```python
from build123d import *

# Parameters (mm, degrees)
SKETCH1_R               = 7.25
SKETCH1_R_2             = 4.25
SKETCH1_W               = 3
SKETCH1_H               = 32
SKETCH1_W_2             = 32
SKETCH1_H_2             = 3
BOSS_EXTRUDE1_DEPTH     = 2
SKETCH1_3_R             = 7.25
SKETCH1_3_R_2           = 4.25
BOSS_EXTRUDE2_DEPTH     = 12
SKETCH5_W               = 9.5
SKETCH5_H               = 6.5
SKETCH5_W_2             = 5.5
SKETCH5_H_2             = 2.5
BOSS_EXTRUDE3_DEPTH     = 10
CUT_EXTRUDE1_DEPTH      = 47.818799643
CUT_EXTRUDE1_DEPTH_BACK = 47.818799643
SKETCH2_R               = 1.5
CUT_EXTRUDE3_DEPTH      = 47.818799643
CUT_EXTRUDE3_DEPTH_BACK = 47.818799643
SKETCH3_R               = 4.25


with BuildPart() as part:
    # Sketch1 → Boss-Extrude1 (new body)
    # profile 1 of 17: a face of its own
    with BuildSketch(Plane(origin=(0, 0, 0), x_dir=(1, 0, 0), z_dir=(0, 1, 0))):
        Circle(SKETCH1_R)
        Circle(SKETCH1_R_2, mode=Mode.SUBTRACT)
    # profile 2 of 17: a face of its own
    with BuildSketch(Plane(origin=(0, 0, 0), x_dir=(1, 0, 0), z_dir=(0, 1, 0))):
        Polygon((-0.461939766, 0.191341716), (11.783930069, 29.755486757), (14.555568667, 28.607436459), (2.309698831, -0.956708581), align=None)
    # profile 3 of 17: a face of its own
    with BuildSketch(Plane(origin=(0, 0, 0), x_dir=(1, 0, 0), z_dir=(0, 1, 0))):
        with Locations((1, 16)):
            Rectangle(SKETCH1_W, SKETCH1_H)
    # profile 4 of 17: a face of its own
    with BuildSketch(Plane(origin=(0, 0, 0), x_dir=(1, 0, 0), z_dir=(0, 1, 0))):
        Polygon((-0.353553391, 0.353553391), (22.273863607, 22.980970389), (24.395183951, 20.859650045), (1.767766953, -1.767766953), align=None)
    # profile 5 of 17: a face of its own
    with BuildSketch(Plane(origin=(0, 0, 0), x_dir=(1, 0, 0), z_dir=(0, 1, 0))):
        Polygon((-0.191341716, 0.461939766), (29.372803324, 12.707809602), (30.520853621, 9.936171004), (0.956708581, -2.309698831), align=None)
    # profile 6 of 17: a face of its own
    with BuildSketch(Plane(origin=(0, 0, 0), x_dir=(1, 0, 0), z_dir=(0, 1, 0))):
        with Locations((16, -1)):
            Rectangle(SKETCH1_W_2, SKETCH1_H_2)
    # profile 7 of 17: a face of its own
    with BuildSketch(Plane(origin=(0, 0, 0), x_dir=(1, 0, 0), z_dir=(0, 1, 0))):
        Polygon((0.191341716, 0.461939766), (29.755486757, -11.783930069), (28.607436459, -14.555568667), (-0.956708581, -2.309698831), align=None)
    # profile 8 of 17: a face of its own
    with BuildSketch(Plane(origin=(0, 0, 0), x_dir=(1, 0, 0), z_dir=(0, 1, 0))):
        Polygon((0.353553391, 0.353553391), (22.980970389, -22.273863607), (20.859650045, -24.395183951), (-1.767766953, -1.767766953), align=None)
    # profile 9 of 17: a face of its own
    with BuildSketch(Plane(origin=(0, 0, 0), x_dir=(1, 0, 0), z_dir=(0, 1, 0))):
        Polygon((0.461939766, 0.191341716), (12.707809602, -29.372803324), (9.936171004, -30.520853621), (-2.309698831, -0.956708581), align=None)
    # profile 10 of 17: a face of its own
    with BuildSketch(Plane(origin=(0, 0, 0), x_dir=(1, 0, 0), z_dir=(0, 1, 0))):
        with Locations((-1, -16)):
            Rectangle(SKETCH1_W, SKETCH1_H)
    # profile 11 of 17: a face of its own
    with BuildSketch(Plane(origin=(0, 0, 0), x_dir=(1, 0, 0), z_dir=(0, 1, 0))):
        Polygon((0.461939766, -0.191341716), (-11.783930069, -29.755486757), (-14.555568667, -28.607436459), (-2.309698831, 0.956708581), align=None)
    # profile 12 of 17: a face of its own
    with BuildSketch(Plane(origin=(0, 0, 0), x_dir=(1, 0, 0), z_dir=(0, 1, 0))):
        Polygon((0.353553391, -0.353553391), (-22.273863607, -22.980970389), (-24.395183951, -20.859650045), (-1.767766953, 1.767766953), align=None)
    # profile 13 of 17: a face of its own
    with BuildSketch(Plane(origin=(0, 0, 0), x_dir=(1, 0, 0), z_dir=(0, 1, 0))):
        Polygon((0.191341716, -0.461939766), (-29.372803324, -12.707809602), (-30.520853621, -9.936171004), (-0.956708581, 2.309698831), align=None)
    # profile 14 of 17: a face of its own
    with BuildSketch(Plane(origin=(0, 0, 0), x_dir=(1, 0, 0), z_dir=(0, 1, 0))):
        with Locations((-16, 1)):
            Rectangle(SKETCH1_W_2, SKETCH1_H_2)
    # profile 15 of 17: a face of its own
    with BuildSketch(Plane(origin=(0, 0, 0), x_dir=(1, 0, 0), z_dir=(0, 1, 0))):
        Polygon((-0.191341716, -0.461939766), (-29.755486757, 11.783930069), (-28.607436459, 14.555568667), (0.956708581, 2.309698831), align=None)
    # profile 16 of 17: a face of its own
    with BuildSketch(Plane(origin=(0, 0, 0), x_dir=(1, 0, 0), z_dir=(0, 1, 0))):
        Polygon((-0.353553391, -0.353553391), (-22.980970389, 22.273863607), (-20.859650045, 24.395183951), (1.767766953, 1.767766953), align=None)
    # profile 17 of 17: a face of its own
    with BuildSketch(Plane(origin=(0, 0, 0), x_dir=(1, 0, 0), z_dir=(0, 1, 0))):
        Polygon((-0.461939766, -0.191341716), (-12.707809602, 29.372803324), (-9.936171004, 30.520853621), (2.309698831, 0.956708581), align=None)
    extrude(amount=BOSS_EXTRUDE1_DEPTH)

    # Sketch1_3 → Boss-Extrude2 (add)
    with BuildSketch(Plane(origin=(0, 0, 0), x_dir=(1, 0, 0), z_dir=(0, 1, 0))):
        with Locations(Location((0, 0, 0), (0, 0, 270))):
            Circle(SKETCH1_3_R)
        with Locations(Location((0, 0, 0), (0, 0, 270))):
            Circle(SKETCH1_3_R_2, mode=Mode.SUBTRACT)
    extrude(amount=BOSS_EXTRUDE2_DEPTH)

    # Sketch5 → Boss-Extrude3 (add)
    with BuildSketch(Plane(origin=(0, 12, 0), x_dir=(1, 0, 0), z_dir=(0, 1, 0))):
        with Locations((0, 8.75)):
            Rectangle(SKETCH5_W, SKETCH5_H)
        with Locations((0, 8.75)):
            Rectangle(SKETCH5_W_2, SKETCH5_H_2, mode=Mode.SUBTRACT)
    extrude(amount=-BOSS_EXTRUDE3_DEPTH)

    # Sketch2 → Cut-Extrude1 (cut, two sides: drawn at the far end of the back side and taken through both)
    with BuildSketch(Plane.XY.offset(-CUT_EXTRUDE1_DEPTH_BACK)):
        with Locations((0, 9)):
            Circle(SKETCH2_R)
    extrude(amount=CUT_EXTRUDE1_DEPTH + CUT_EXTRUDE1_DEPTH_BACK, mode=Mode.SUBTRACT)

    # Sketch3 → Cut-Extrude3 (cut, two sides: drawn at the far end of the back side and taken through both)
    with BuildSketch(Plane(origin=(0, 12, 0), x_dir=(1, 0, 0), z_dir=(0, 1, 0)).offset(-CUT_EXTRUDE3_DEPTH_BACK)):
        with Locations(Location((0, 0, 0), (0, 0, 270))):
            Circle(SKETCH3_R)
    extrude(amount=CUT_EXTRUDE3_DEPTH + CUT_EXTRUDE3_DEPTH_BACK, mode=Mode.SUBTRACT)


solid = part.part
```
Here's how the part is built. I have some questions about the finished solid (model axes, mm). A direction names the side the tool comes from. Coordinates: 2 decimals unless noted, no trailing zeros. One line per item, written item: value.
1) We'd pull the mould along X, two halves only. Please class faces 6 (the flat face through (4.75, 7, -9)), 7 (the flat face through (-29.94, 0.99, 11.34)), 8 (the flat face through (7.077, 0.986, -18.392)): pulls with the +X half, pulls with the -X half, needs draft (parallel to the pull), parting line crosses it, or undercut.
Model answer:
face 6: pulls with the +X half
face 7: pulls with the -X half
face 8: undercut
2) Suppose I cut it at A-A on y = 3.25. State how many separate pieces and enclosed holes the cut face has, and give its area (3 significant figures).
Model answer:
separate pieces: 1
enclosed holes: 2
area: 145 mm²
3) I'm going to push flat-ended pins straight in: P1, Ø0.8, axis at y = 9.5, z = -9.5, coming from the -X side; P2, Ø4, axis at x = 0, y = 9, coming from the -Z side; P3, Ø2, axis at y = 8, z = -8, coming from the +X side; P4, Ø2, axis at x = 3, z = -9.5, coming from the -Y side. Where does each tip first touch, or does it pass through?
Model answer:
P1: stops at x = -4.75
P2: stops at z = -12
P3: stops at x = 4.75
P4: stops at y = 0
4) I need wall thicknesses on line 1 along Z through (x, y) = (0, 4.5); line 2 along X through (y, z) = (6, 0); line 3 along X through (y, z) = (3.25, -8). Which ranges of each line are inside material? Lowest first, please.
Model answer:
line 1: z = -12 to -10, -7.5 to -4.25, 4.25 to 7.25
line 2: x = -7.25 to -4.25, 4.25 to 7.25
line 3: x = -4.75 to -2.75, 2.75 to 4.75
5) On a 3-axis mill with a long thin cutter (end or side, diameter ignored), from which of +Z, -Z, +X, -X, +Y, -Y can I reach the whole of each face in a straight line? I mean faces 1 (the cylindrical face through (1.386, 8.425, -5.763)), 2 (the flat face through (-18.392, 0.986, -7.077)), 3 (the flat face through (-15.799, 0.986, 12.264)), 4 (the flat face through (1, 2, -22)), 5 (the flat face through (18.392, 0.986, 7.077)). Say none if no direction works.
Model answer:
face 1: +Z, -Z
face 2: -X, +Y, -Y
face 3: +Y, -Y
face 4: -Z, +X, -X, +Y
face 5: +X, +Y, -Y
